```python
from build123d import *

# Parameters (mm, degrees)
EXTRUDE_1_DEPTH        = 1.25
EXTRUDE_2_DEPTH        = 0.5
FILLET_1_R             = 2
FILLET_1_OF_MIRROR_1_R = 2
FILLET_2_R             = 0.2
CHAMFER_1_SIZE         = 0.2
CHAMFER_1_SIZE2        = 0.15168085


with BuildPart() as part:
    # Sketch 1 → Revolve 1 (revolve)
    with BuildSketch(Plane.XY, mode=Mode.PRIVATE) as revolve_1_sk:
        Polygon((6, 0), (6, 2.5), (7, 2.5), (7, 3), (5.5, 9.4), (3.5, 9.4), (5, 6), (5, 0), align=None)
    revolve(revolve_1_sk.sketch.rotate(Axis((0, 0, 0), (0, 1, 0)), 90), axis=Axis((0, 0, 0), (0, 1, 0)))

    # Sketch 2 → Extrude 1 (add, symmetric)
    with BuildSketch(Plane(origin=(0, 0, 0), x_dir=(0, 0, -1), z_dir=(1, 0, 0))):
        Polygon((-7, 3), (-12.5, 3), (-11.7185832, 7.431634889), (-5.614095661, 8.913191845), (-5, 9.062232643), (-5, 3), align=None)
    extrude_1 = extrude(amount=EXTRUDE_1_DEPTH, both=True)

    # Sketch 3 → Extrude 2 (add)
    with BuildSketch(Plane.XZ.offset(-3)):
        with BuildLine():
            Line((-0.5, 7.5), (-0.5, 6.982120022))
            ThreePointArc((-0.5, 6.982120022), (0, 7), (0.5, 6.982120022))
            Line((0.5, 6.982120022), (0.5, 7.5))
            ThreePointArc((0.5, 7.5), (0, 8), (-0.5, 7.5))
        make_face()
    extrude_2 = extrude(amount=EXTRUDE_2_DEPTH)

    # Fillet 1
    fillet_1_edges = [part.edges().sort_by_distance(p)[0] for p in [
        (0, 7.431634889, 11.7185832),
    ]]
    fillet(fillet_1_edges, radius=FILLET_1_R)

    # Mirror 1: Extrude 1, Extrude 2 across plane
    add(extrude_1.mirror(Plane.XY))
    add(extrude_2.mirror(Plane.XY))

    # Fillet 1 of Mirror 1
    fillet_1_of_mirror_1_edges = [part.edges().sort_by_distance(p)[0] for p in [
        (0, 7.431634889, -11.7185832),
    ]]
    fillet(fillet_1_of_mirror_1_edges, radius=FILLET_1_OF_MIRROR_1_R)

    # Fillet 2
    fillet_2_edges = [part.edges().sort_by_distance(p)[0] for p in [
        (-1.25, 4.571891442, -12.222833128),
        (-1.25, 7.165047592, -11.434488481),
        (1.25, 4.571891442, -12.222833128),
        (1.25, 7.165047592, -11.434488481),
        (-1.25, 4.571891442, 12.222833128),
        (-1.25, 7.165047592, 11.434488481),
        (1.25, 4.571891442, 12.222833128),
        (1.25, 7.165047592, 11.434488481),
        (-1.25, 8.344789205, -7.956095957),
        (1.25, 8.344789205, -7.956095957),
        (-1.25, 8.344789205, 7.956095957),
        (1.25, 8.344789205, 7.956095957),
        (0, 9.4, 5.5),
    ]]
    fillet(fillet_2_edges, radius=FILLET_2_R)

    # Chamfer 1
    chamfer_1_edges = [part.edges().sort_by_distance(p)[0] for p in [
        (0, 9.4, 3.5),
    ]]
    chamfer_1_side = [part.faces().sort_by_distance(p)[0] for p in [
        (0, 7.7, 4.25),
    ]]
    chamfer(chamfer_1_edges, length=CHAMFER_1_SIZE, length2=CHAMFER_1_SIZE2, reference=chamfer_1_side[0])


solid = part.part
```
CAD build for the part. Positions are in the model's coordinates, mm. A direction names the side the tool comes from. Coordinates: 2 decimals unless noted, no trailing zeros. Order: outer loops, then holes, each group sorted by start corner. A loop starts at its lowest first (then second) coordinate and runs counter-clockwise, first axis right, second up. Notation, with made-up numbers: (51, 75) - (58, 75) arc R20 ccw to (58, 108) - close; hole circle Ø5 at (-40, -2.5). An arc over 180 degrees is marked (long way). Answer in a Markdown table with one row per item.
1. Drill centre lines: L1, parallel to X at y = 1.7, z = 0; L2, parallel to X at y = 8.25, z = -0.25; L3, parallel to X at y = 4.25, z = 10. Where is each one in solid material? Low to high. Write a range as from..to.
Answer:
| item | result |
|---|---|
| L1 | -6..-5, 5..6 |
| L2 | -5.76..-4, 4..5.76 |
| L3 | -1.25..1.25 |
2. Slice it at B-B, the plane y = 1.5. List the corners of the cut face in (x, z).
Answer:
| item | result |
|---|---|
| outline | circle Ø12 at (0, 0); hole circle Ø10 at (0, 0) |
3. 3-axis set-ups, long thin cutter, end or side, ignore diameter. For faces 1 (the face through (-6, 2.5, -2)), 2 (the face through (1.25, 6, -9)), 3 (the face through (-1.25, 6, 9)): which of +Z, -Z, +X, -X, +Y, -Y reach the whole face in a straight line?
Answer:
| item | result |
|---|---|
| face 1 | -Y |
| face 2 | -Z, +X, +Y |
| face 3 | +Z, -X, +Y |
4. Pull direction X, two halves, no side cores. Call faces 4 (the face through (0, 3, 5)), 5 (the face through (-1.25, 6, -9)), 6 (the face through (-1.78, 7.55, -5.66)): +X half, -X half, draft (parallel to the pull), parting line (faces both ways), or undercut.
Answer:
| item | result |
|---|---|
| face 4 | undercut |
| face 5 | -X half |
| face 6 | parting line |
5. Slice it at A-A, the plane z = 0. List the corners of the cut face in (x, y), then the cut area to 3 significant figures.
Answer:
| item | result |
|---|---|
| outline | (-7, 2.5) - (-6, 2.5) - (-6, 0) - (-5, 0) - (-5, 6) - (-3.58, 9.22) - (-3.65, 9.4) - (-5.34, 9.4) arc R0.2 ccw to (-5.54, 9.25) - (-7, 3) - close; (3.58, 9.22) - (5, 6) - (5, 0) - (6, 0) - (6, 2.5) - (7, 2.5) - (7, 3) - (5.54, 9.25) arc R0.2 ccw to (5.34, 9.4) - (3.65, 9.4) - close |
| area | 28.1 mm² |
6. Flat gauge pins, fed straight in: P1, Ø2, axis at x = 0.5, z = 9, coming from the -Y side; P2, Ø3, axis at y = 5, z = -9.5, coming from the +X side; P3, Ø1, axis at x = 4, z = -8, coming from the +Y side; P4, Ø7, axis at x = 1, z = 1, coming from the -Y side. Where does each tip first touch, or does it go through?
Answer:
| item | result |
|---|---|
| P1 | y = 3 |
| P2 | x = 1.25 |
| P3 | through |
| P4 | y = 6.19 |
